Verification items for the finished model (mm, model axes). A direction names the side the tool comes from. Coordinates: 2 decimals unless noted, no trailing zeros. Order: outer loops, then holes, each group sorted by start corner. A loop starts at its lowest first (then second) coordinate and runs counter-clockwise, first axis right, second up. Notation, with made-up numbers: M 69.25,41 L 82.25,41 A28 ccw 82.25,72 Z; hole C -28.5,41 d3. An arc over 180 degrees is marked long. Return JSON: item names as keys, results as strings.
```python
from build123d import *

# Parameters (mm, degrees)
MAIN_DEPTH            = 2.5
ESQUISSE2_R           = 2.5
ORIGINALBRACKET_DEPTH = 2
CUT_EXTRUDE1_DEPTH    = 3


with BuildPart() as part:
    # Esquisse1 → Main (new body)
    with BuildSketch(Plane.XY):
        with BuildLine():
            Line((0, 10), (62, 10))
            ThreePointArc((62, 10), (72, 0), (62, -10))
            Line((62, -10), (0, -10))
            ThreePointArc((0, -10), (-10, 0), (0, 10))
        make_face()
        with BuildLine():
            Line((0.349090909, 3.583034404), (16.693939394, 1.990574669))
            ThreePointArc((16.693939394, 1.990574669), (18.5, 0), (16.693939394, -1.990574669))
            Line((16.693939394, -1.990574669), (0.349090909, -3.583034404))
            ThreePointArc((0.349090909, -3.583034404), (-3.6, 0), (0.349090909, 3.583034404))
        make_face(mode=Mode.SUBTRACT)
        with BuildLine():
            Line((27, 5.3), (62, 5.3))
            ThreePointArc((62, 5.3), (67.3, 0), (62, -5.3))
            Line((62, -5.3), (27, -5.3))
            ThreePointArc((27, -5.3), (21.7, 0), (27, 5.3))
        make_face(mode=Mode.SUBTRACT)
    extrude(amount=MAIN_DEPTH)

    # Esquisse2 → OriginalBracket (add)
    with BuildSketch(Plane(origin=(0, 0, 0), x_dir=(-1, 0, 0), z_dir=(0, 0, -1))):
        with BuildLine():
            Line((0, -10), (-62, -10))
            ThreePointArc((-62, -10), (-72, 0), (-62, 10))
            Line((-62, 10), (0, 10))
            ThreePointArc((0, 10), (10, 0), (0, -10))
        make_face()
        Circle(ESQUISSE2_R, mode=Mode.SUBTRACT)
    extrude(amount=ORIGINALBRACKET_DEPTH)

    # Sketch1 → Cut-Extrude1 (cut, through all)
    with BuildSketch(Plane.XY):
        with BuildLine():
            Line((27, 5.3), (62, 5.3))
            ThreePointArc((62, 5.3), (67.3, 0), (62, -5.3))
            Line((62, -5.3), (27, -5.3))
            ThreePointArc((27, -5.3), (21.7, 0), (27, 5.3))
        make_face()
    extrude(amount=-CUT_EXTRUDE1_DEPTH, mode=Mode.SUBTRACT)


solid = part.part
```
Q1. Material ranges on line 1 along X through (y, z) = (0, 1.8); line 2 along Y through (x, z) = (0, -1.05); line 3 along Y through (x, z) = (0, 0.8), recorded low to high.
Values:
{"line 1": "-10 to -3.6, 18.5 to 21.7, 67.3 to 72", "line 2": "-10 to -2.5, 2.5 to 10", "line 3": "-10 to -3.6, 3.6 to 10"}
Q2. Go/stop test with flat-tipped pins: pin 1 (2 mm diameter, centred on x = 12, y = 1, fed in from +Z); pin 2 (4.5 mm diameter, centred on x = 0, y = 0, fed in from -Z). Record where each tip stops, or that it passes through.
Values:
{"pin 1": "z = 0", "pin 2": "through"}
Q3. Draft check along X on faces 1 (the face through (32, 7, 2.5)), 2 (the face through (21.7, -0.1, 0.3)), 3 (the face through (72, 0, 0)), 4 (the face through (67.3, 0.1, 0.3)). Enter one of: pulls with the +X half, pulls with the -X half, needs draft (parallel to the pull), parting line crosses it, or undercut.
Values:
{"face 1": "needs draft", "face 2": "undercut", "face 3": "pulls with the +X half", "face 4": "undercut"}
Q4. Cross-section at C-C, the plane z = 1.1. Record the boundary of the cut face in (x, y), and give its area (3 significant figures).
Values:
{"outline": "M 0,-10 L 62,-10 A10 ccw 62,10 L 0,10 A10 ccw Z; hole M 0.35,-3.58 L 16.69,-1.99 A2 ccw 16.69,1.99 L 0.35,3.58 A3.6 ccw long Z; hole M 27,-5.3 L 62,-5.3 A5.3 ccw 62,5.3 L 27,5.3 A5.3 ccw Z", "area": "975 mm^2"}
Q5. Cross-section at D-D, the plane x = 10. Record the boundary of the cut face in (y, z), and give its area (3 significant figures).
Values:
{"outline": "M -10,-2 L 10,-2 L 10,2.5 L 2.64,2.5 L 2.64,0 L -2.64,0 L -2.64,2.5 L -10,2.5 Z", "area": "76.8 mm^2"}
Q6. Cross-section at B-B, the plane x = 34. Record the boundary of the cut face in (y, z).
Values:
{"outline": "M -10,-2 L -5.3,-2 L -5.3,2.5 L -10,2.5 Z; M 5.3,-2 L 10,-2 L 10,2.5 L 5.3,2.5 Z"}
Q7. Cross-section at A-A, the plane y = 0. Record the boundary of the cut face in (x, z).
Values:
{"outline": "M -10,-2 L -2.5,-2 L -2.5,0 L -3.6,0 L -3.6,2.5 L -10,2.5 Z; M 2.5,-2 L 21.7,-2 L 21.7,2.5 L 18.5,2.5 L 18.5,0 L 2.5,0 Z; M 67.3,-2 L 72,-2 L 72,2.5 L 67.3,2.5 Z"}
Q8. Tool access check on faces 5 (the face through (-3.6, -0.1, 1.2)), 6 (the face through (45, -5.3, 0)), 7 (the face through (21, 0, -2)). Record the directions out of +Z, -Z, +X, -X, +Y, -Y that give a thin tool (end or side, any length) a straight path to the whole face; none if there is none.
Values:
{"face 5": "+Z", "face 6": "+Z, -Z", "face 7": "-Z, +X, -X, +Y, -Y"}
